For this review, take the finished solid that the model builds, in its own axes (mm). Coordinates: 2 decimals unless noted, no trailing zeros. Write each loop counter-clockwise with the first axis right and the second up, starting at its lowest first coordinate (ties: lowest second). Pieces come first, ordered by that corner, then holes. Notation, with made-up numbers: (-2, 86) - (52, 86) arc R16 ccw to (52, 93) - close; hole circle Ø9 at (73.5, 83.25). An arc over 180 degrees is marked (long way). Write each question's results on one line, items separated by ' | '.
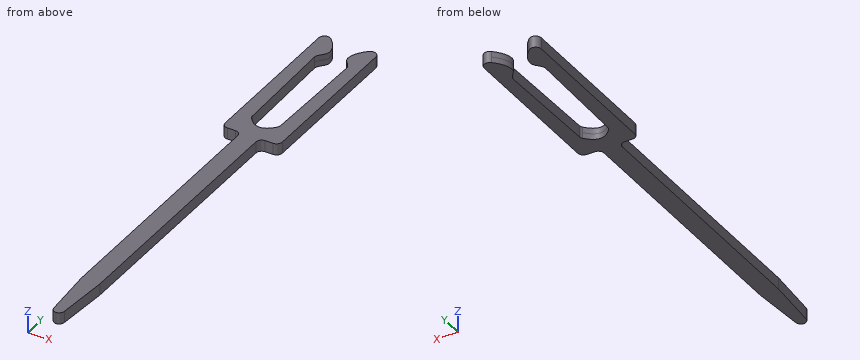
from build123d import *

# Parameters (mm, degrees)
BOSS_EXTRUDE1_DEPTH = 0.2


with BuildPart() as part:
    # Sketch1 → Boss-Extrude1 (new body, symmetric)
    with BuildSketch(Plane.XY):
        with BuildLine():
            Line((-0.32, -7.733224852), (-0.32, 1.266775148))
            ThreePointArc((-0.32, 1.266775148), (-0.378578644, 1.408196504), (-0.52, 1.466775148))
            Line((-0.52, 1.466775148), (-0.8, 1.466775148))
            ThreePointArc((-0.8, 1.466775148), (-0.941421356, 1.525353792), (-1, 1.666775148))
            Line((-1, 1.666775148), (-1, 7.057198685))
            ThreePointArc((-1, 7.057198685), (-0.87939743, 7.240763518), (-0.663039519, 7.202944445))
            add(Edge.make_bspline(
                [(-0.663039519, 7.202944445), (-0.487599251, 7.038079386), (-0.326177604, 6.816155039), (-0.310671132, 6.388247389), (-0.548453888, 6.275984696), (-0.567669208, 6.108344969)],
                knots=[0.253308427, 0.253308427, 0.253308427, 0.253308427, 0.663171976, 0.707067436, 1, 1, 1, 1], degree=3))
            Line((-0.567669208, 6.108344969), (-0.495215905, 2.401684718))
            ThreePointArc((-0.495215905, 2.401684718), (-0.483221967, 2.337269967), (-0.451053839, 2.280188217))
            add(Edge.make_bspline(
                [(-0.451053839, 2.280188217), (0, 1.719811783), (0.451053839, 2.280188217)],
                knots=[0.043404734, 0.043404734, 0.043404734, 0.956595266, 0.956595266, 0.956595266], degree=2))
            ThreePointArc((0.451053839, 2.280188217), (0.483221967, 2.337269967), (0.495215905, 2.401684718))
            Line((0.495215905, 2.401684718), (0.567669208, 6.108344969))
            add(Edge.make_bspline(
                [(0.663039519, 7.202944445), (0.487599251, 7.038079386), (0.326177604, 6.816155039), (0.310671132, 6.388247389), (0.548453888, 6.275984696), (0.567669208, 6.108344969)],
                knots=[0.253308427, 0.253308427, 0.253308427, 0.253308427, 0.663171976, 0.707067436, 1, 1, 1, 1], degree=3))
            ThreePointArc((0.663039519, 7.202944445), (0.87939743, 7.240763518), (1, 7.057198685))
            Line((1, 7.057198685), (1, 1.666775148))
            ThreePointArc((1, 1.666775148), (0.941421356, 1.525353792), (0.8, 1.466775148))
            Line((0.8, 1.466775148), (0.52, 1.466775148))
            ThreePointArc((0.52, 1.466775148), (0.378578644, 1.408196504), (0.32, 1.266775148))
            Line((0.32, 1.266775148), (0.32, -7.733224852))
            Line((0.32, -7.733224852), (0.183878151, -9.548182842))
            ThreePointArc((0.183878151, -9.548182842), (0.126073555, -9.674431974), (0, -9.732618516))
            ThreePointArc((0, -9.732618516), (-0.126073555, -9.674431974), (-0.183878151, -9.548182842))
            Line((-0.183878151, -9.548182842), (-0.32, -7.733224852))
        make_face()
    extrude(amount=BOSS_EXTRUDE1_DEPTH, both=True)


solid = part.part
Q1. Take a section at A-A on y = 4.25. State the section outline as (x, z) points, plus the area to 3 significant figures.
Results found:
outline: (-1, -0.2) - (-0.53, -0.2) - (-0.53, 0.2) - (-1, 0.2) - close; (0.53, -0.2) - (1, -0.2) - (1, 0.2) - (0.53, 0.2) - close | area: 0.375 mm2
Q2. Take a section at B-B on y = -3.5. State the section outline as (x, z) points.
Results found:
outline: (-0.32, -0.2) - (0.32, -0.2) - (0.32, 0.2) - (-0.32, 0.2) - close
Q3. Wall thickness on line 1 along X through (y, z) = (3.75, 0); line 2 along X through (y, z) = (6, 0); line 3 along X through (y, z) = (-0.5, -0.05): over which ranges is each line inside the solid? List them lowest first. Write a range as from..to.
Results found:
line 1: -1..-0.52, 0.52..1 | line 2: -1..-0.57, 0.57..1 | line 3: -0.32..0.32
